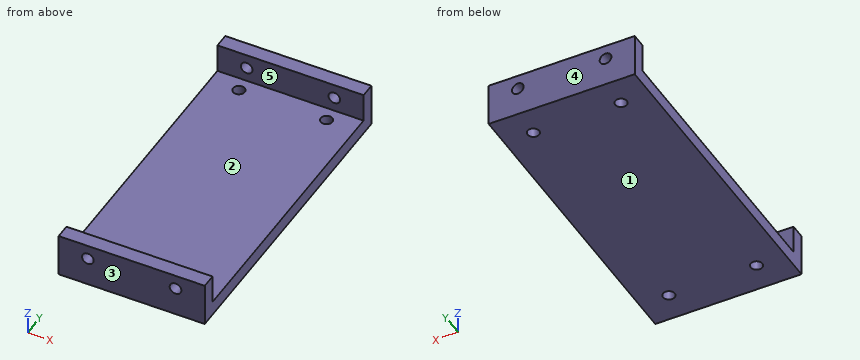
```python
from build123d import *

# Parameters (mm, degrees)
SKETCH1_W                       = 50
SKETCH1_H                       = 15
BOSS_EXTRUDE1_DEPTH             = 5
SKETCH2_W                       = 50
SKETCH2_H                       = 5
BOSS_EXTRUDE2_DEPTH             = 97
SKETCH3_W                       = 50
SKETCH3_H                       = 15
BOSS_EXTRUDE3_DEPTH             = 5
F_4_0MM_DOWEL_HOLE1_D           = 4
F_4_0MM_DOWEL_HOLE1_ON_FACE_2_D = 4
F_4_0MM_DOWEL_HOLE1_ON_FACE_3_D = 4


with BuildPart() as part:
    # Sketch1 → Boss-Extrude1 (new body)
    with BuildSketch(Plane(origin=(0, 0, 0), x_dir=(1, 0, 0), z_dir=(0, 1, 0))):
        Rectangle(SKETCH1_W, SKETCH1_H)
    extrude(amount=-BOSS_EXTRUDE1_DEPTH)

    # Sketch2 → Boss-Extrude2 (add)
    with BuildSketch(Plane(origin=(0, 0, 0), x_dir=(1, 0, 0), z_dir=(0, 1, 0))):
        with Locations((0, 5)):
            Rectangle(SKETCH2_W, SKETCH2_H)
    extrude(amount=BOSS_EXTRUDE2_DEPTH)

    # Sketch3 → Boss-Extrude3 (add)
    with BuildSketch(Plane(origin=(0, 97, 0), x_dir=(1, 0, 0), z_dir=(0, 1, 0))):
        Rectangle(SKETCH3_W, SKETCH3_H)
    extrude(amount=BOSS_EXTRUDE3_DEPTH)

    # Ø4.0mm Dowel Hole1 (through all)
    with Locations(Plane(origin=(-15, 0, 2.5), x_dir=(0, 0, 1), z_dir=(0, 1, 0))):
        with Locations((0, 0), (0, 30)):
            Hole(F_4_0MM_DOWEL_HOLE1_D / 2)

    # Ø4.0mm Dowel Hole1 on face 2 (through all)
    with Locations(Plane(origin=(-15, 5, -2.5), x_dir=(1, 0, 0), z_dir=(0, 0, 1))):
        with Locations((0, 0), (30, 0), (0, 87), (30, 87)):
            Hole(F_4_0MM_DOWEL_HOLE1_ON_FACE_2_D / 2)

    # Ø4.0mm Dowel Hole1 on face 3 (through all)
    with Locations(Plane(origin=(15, 97, 2.5), x_dir=(0, 0, -1), z_dir=(0, -1, 0))):
        with Locations((0, 0), (0, -30)):
            Hole(F_4_0MM_DOWEL_HOLE1_ON_FACE_3_D / 2)


solid = part.part
```
The model under review builds one solid part; all positions refer to its coordinate system, in mm. Face numbers are marked on the shaded views. A direction names the side the tool comes from. Give positions to 0.01 mm unless a question says otherwise; leave off trailing zeros. Write each loop counter-clockwise with the first axis right and the second up, starting at its lowest first coordinate (ties: lowest second). Pieces come first, ordered by that corner, then holes. Notation, with made-up numbers: (-10.5, 25) - (11.5, 25) arc R4 cw to (11.5, 29) - close; hole circle Ø3 at (60.25, 51.25). An arc over 180 degrees is marked (long way). Answer in a Markdown table with one row per item. Add a question column.
1. Insertion check: P1, Ø2.5, axis at x = 15, y = 92, coming from the +Z side; P2, Ø4.5, axis at x = -15, y = 5, coming from the +Z side. Each pin has a flat end and moves straight along its axis. Give the tip position at first contact, or say it passes through.
2. Tool access review of the marked faces 1 and 2: name each direction out of +Z, -Z, +X, -X, +Y, -Y from which nothing blocks a thin tool from reaching the whole face with its end or side.
3. We need section D-D on y = 37. Write out the cut boundary in (x, z), then the cut area to 3 significant figures.
4. We need section B-B on x = 18. Write out the cut boundary in (y, z), then the cut area to 3 significant figures.
5. Draft analysis for pull direction Y (two halves, no side actions). For the marked faces 3, 4 and 5, state which applies: +Y half, -Y half, draft (parallel to the pull), parting line (faces both ways), or undercut.
6. Wall thickness on line 1 along X through (y, z) = (101, 2.5); line 2 along Y through (x, z) = (-15, -3.7); line 3 along Z through (x, y) = (-15, -2): over which ranges is each line inside the solid? List them lowest first. Write a range as [from, to].
7. We need section C-C on x = -15. Write out the cut boundary in (y, z), then the cut area to 3 significant figures.
8. We need section A-A on z = 2.5. Write out the cut boundary in (x, y), then the cut area to 3 significant figures.
Ans:
| question | item | result |
|---|---|---|
| 1 | P1 | passes through |
| 1 | P2 | stops at z = -2.5 |
| 2 | face 1 | -Z, +X, -X, +Y, -Y |
| 2 | face 2 | +Z, +X, -X |
| 3 | outline | (-25, -7.5) - (25, -7.5) - (25, -2.5) - (-25, -2.5) - close |
| 3 | area | 250 mm^2 |
| 4 | outline | (-5, -7.5) - (102, -7.5) - (102, 7.5) - (97, 7.5) - (97, -2.5) - (0, -2.5) - (0, 7.5) - (-5, 7.5) - close |
| 4 | area | 635 mm^2 |
| 5 | face 3 | -Y half |
| 5 | face 4 | +Y half |
| 5 | face 5 | undercut |
| 6 | line 1 | x = [-25, -17], [-13, 13], [17, 25] |
| 6 | line 2 | y = [-5, 3], [7, 90], [94, 102] |
| 6 | line 3 | z = [-7.5, 0.5], [4.5, 7.5] |
| 7 | outline | (-5, -7.5) - (3, -7.5) - (3, -2.5) - (0, -2.5) - (0, 0.5) - (-5, 0.5) - close; (-5, 4.5) - (0, 4.5) - (0, 7.5) - (-5, 7.5) - close; (7, -7.5) - (90, -7.5) - (90, -2.5) - (7, -2.5) - close; (94, -7.5) - (102, -7.5) - (102, 0.5) - (97, 0.5) - (97, -2.5) - (94, -2.5) - close; (97, 4.5) - (102, 4.5) - (102, 7.5) - (97, 7.5) - close |
| 7 | area | 555 mm^2 |
| 8 | outline | (-25, -5) - (-17, -5) - (-17, 0) - (-25, 0) - close; (-25, 97) - (-17, 97) - (-17, 102) - (-25, 102) - close; (-13, -5) - (13, -5) - (13, 0) - (-13, 0) - close; (-13, 97) - (13, 97) - (13, 102) - (-13, 102) - close; (17, -5) - (25, -5) - (25, 0) - (17, 0) - close; (17, 97) - (25, 97) - (25, 102) - (17, 102) - close |
| 8 | area | 420 mm^2 |
